Check sheet for the modelled part. Datum: model origin and axes. Units: mm. A direction names the side the tool comes from. Give positions to 0.01 mm unless a question says otherwise; leave off trailing zeros. Order: outer loops, then holes, each group sorted by start corner. A loop starts at its lowest first (then second) coordinate and runs counter-clockwise, first axis right, second up. Notation, with made-up numbers: (3.5, 49.25) - (41.5, 49.25) arc R18 cw to (41.5, 67.25) - close; hole circle Ø11 at (48, 67.25). An arc over 180 degrees is marked (long way). Answer in a Markdown table with one row per item.
from build123d import *

# Parameters (mm, degrees)
F0_W     = 103.156984
F0_H     = 82.587916
F1_DEPTH = 25.4
F3_DEPTH = 25.4
F4_R     = 25.4
F5_DEPTH = 127


with BuildPart() as f1:
    # F0 (on Front) → F1 (new body)
    with BuildSketch(Plane.XZ):
        with Locations((4.793879, -9.056745)):
            Rectangle(F0_W, F0_H)
    extrude(amount=-F1_DEPTH)

    # F2 (on face) → F3 (join)
    with BuildSketch(Plane.XZ):
        Polygon((-8.684613, 32.237213), (-46.784613, 32.237213), (-46.784613, -50.350703), (42.115387, -50.350703), align=None)
    extrude(amount=F3_DEPTH)

    # F4 (on face) → F5 (cut)
    with BuildSketch(Plane(origin=(0, 25.4, 0), x_dir=(-1, 0, 0), z_dir=(0, 1, 0))):
        with Locations((-4.793879, -9.056745)):
            Circle(F4_R)
    extrude(amount=-F5_DEPTH, mode=Mode.SUBTRACT)


solid = f1.part
(1) Access from +Z, -Z, +X, -X, +Y, -Y to the whole of each face (thin tool, end or side, straight path). Record for faces 1 (the flat face through (-23, -25.4, -18)), 2 (the flat face through (33.993, -12.522, -37.147)).
Geometry says:
| item | result |
|---|---|
| face 1 | +Z, -Z, +X, -X, -Y |
| face 2 | +Z, +X, -Y |
(2) Mould release check, pull along X, two halves, no side actions. Record for faces 3 (the cylindrical face through (-18.669, 0.356, -18.785)), 4 (the flat face through (4, 0, -50.351)), 5 (the flat face through (-3.65, -12.52, 24.05)): pulls with the +X half, pulls with the -X half, needs draft (parallel to the pull), parting line crosses it, or undercut.
Geometry says:
| item | result |
|---|---|
| face 3 | undercut |
| face 4 | needs draft |
| face 5 | pulls with the +X half |
(3) Thickness scan on L1, parallel to Y at x = 51, z = -15; L2, parallel to Z at x = -8.5, y = 22.5; L3, parallel to Z at x = 4, y = -22. Record the ranges inside material, lowest first.
Geometry says:
| item | result |
|---|---|
| L1 | 0 to 25.4 |
| L2 | -50.35 to -30.7, 12.59 to 32.24 |
| L3 | -50.35 to -34.44 |
(4) Cross-section at A-A, the plane x = 0. Record the cut outline in (y, z).
Geometry says:
| item | result |
|---|---|
| outline | (-25.4, -50.35) - (25.4, -50.35) - (25.4, -34) - (-25.4, -34) - close; (-25.4, 15.89) - (25.4, 15.89) - (25.4, 32.24) - (0, 32.24) - (0, 18.12) - (-25.4, 18.12) - close |
(5) Cross-section at D-D, the plane x = 18. Record the cut outline in (y, z).
Geometry says:
| item | result |
|---|---|
| outline | (-25.4, -50.35) - (25.4, -50.35) - (25.4, -30.75) - (-25.4, -30.75) - close; (0, 12.64) - (25.4, 12.64) - (25.4, 32.24) - (0, 32.24) - close |
(6) Cross-section at B-B, the plane z = -19. Record the cut outline in (x, y).
Geometry says:
| item | result |
|---|---|
| outline | (-46.78, -25.4) - (-18.58, -25.4) - (-18.58, 25.4) - (-46.78, 25.4) - close; (28.17, 0) - (56.37, 0) - (56.37, 25.4) - (28.17, 25.4) - close |
(7) Gauge pin test, flat ends, axial feed: P1, Ø2, axis at x = 37.5, z = -28.5, coming from the -Y side; P2, Ø6, axis at x = 22.5, y = -19, coming from the +Z side. Record the tip position at first contact, or that the pin passes through.
Geometry says:
| item | result |
|---|---|
| P1 | y = 0 |
| P2 | z = -23.77 |
(8) Cross-section at C-C, the plane y = -10.5. Record the cut outline in (x, z), then the cut area to 3 significant figures.
Geometry says:
| item | result |
|---|---|
| outline | (-46.78, -50.35) - (42.12, -50.35) - (25.64, -23.57) arc R25.4 cw (long way) to (1.25, 16.09) - (-8.68, 32.24) - (-46.78, 32.24) - close |
| area | 3,730 mm² |
